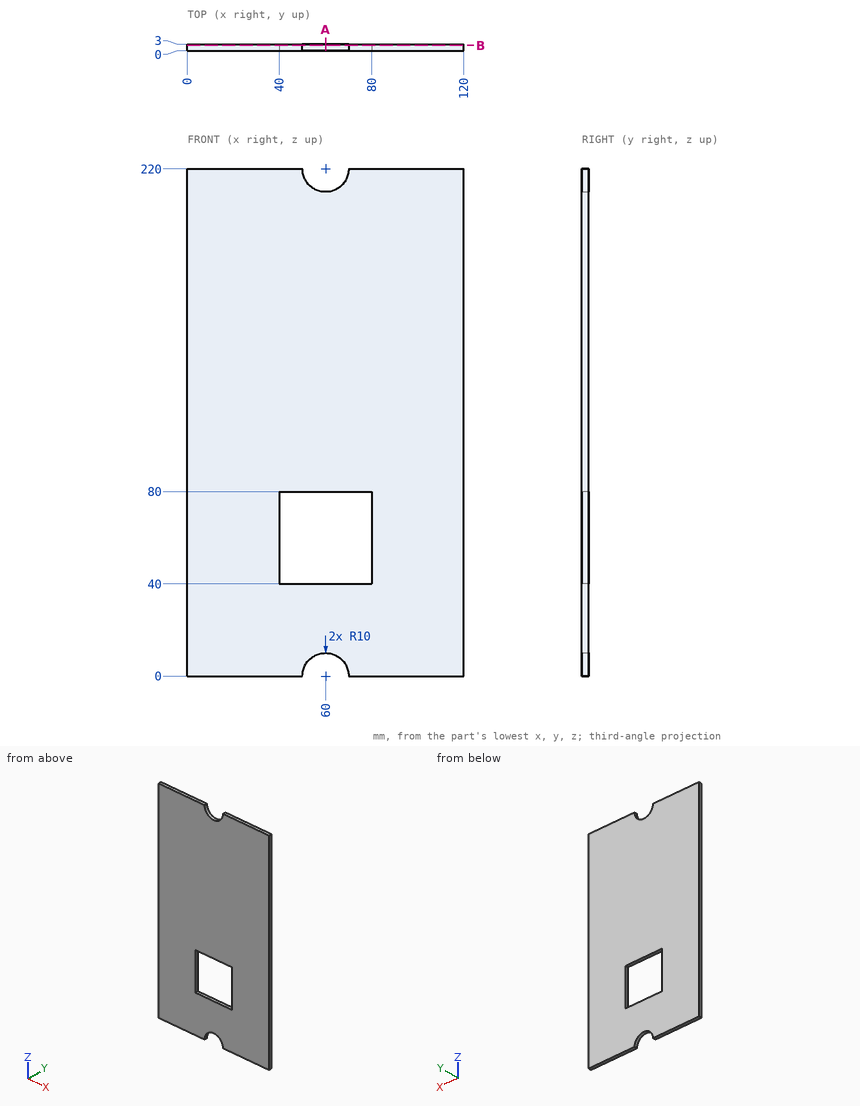
The figure shows three views and two pictorial views of one solid part (mm, origin at its lowest corner). Answer the questions. Coordinates: 2 decimals unless noted, no trailing zeros. Order: outer loops, then holes, each group sorted by start corner. A loop starts at its lowest first (then second) coordinate and runs counter-clockwise, first axis right, second up.
Q1. Consider line 1 (Z direction, x = 59, y = 1.4); line 2 (X direction, y = 2.55, z = 79); line 3 (Z direction, x = 68, y = 2.75). Determine where each line is inside the solid, lowest interval first.
Q2. Given P1, Ø1.5, axis at x = 52.5, y = 1, coming from the -Z side; P2, Ø1.5, axis at x = 59, y = 2, coming from the +Z side, each flat-ended and moving along its own axis, determine where each tip first touches the part or whether it passes through.
Q3. A cutting plane is placed at B-B, the plane y = 2.4. Write down the section's boundary in (x, z).
Q4. A cutting plane is placed at A-A, the plane x = 60. Write down the section's boundary in (y, z).
Answers follow:
1. line 1: z = 9.95 to 40, 80 to 210.05
1. line 2: x = 0 to 40, 80 to 120
1. line 3: z = 6 to 40, 80 to 214
2. P1: stops at z = 5.65
2. P2: stops at z = 210.15
3. outline: (0, 0) - (50, 0) arc R10 cw to (70, 0) - (120, 0) - (120, 220) - (70, 220) arc R10 cw to (50, 220) - (0, 220) - close; hole (40, 40) - (80, 40) - (80, 80) - (40, 80) - close
4. outline: (0, 10) - (3, 10) - (3, 40) - (0, 40) - close; (0, 80) - (3, 80) - (3, 210) - (0, 210) - close
